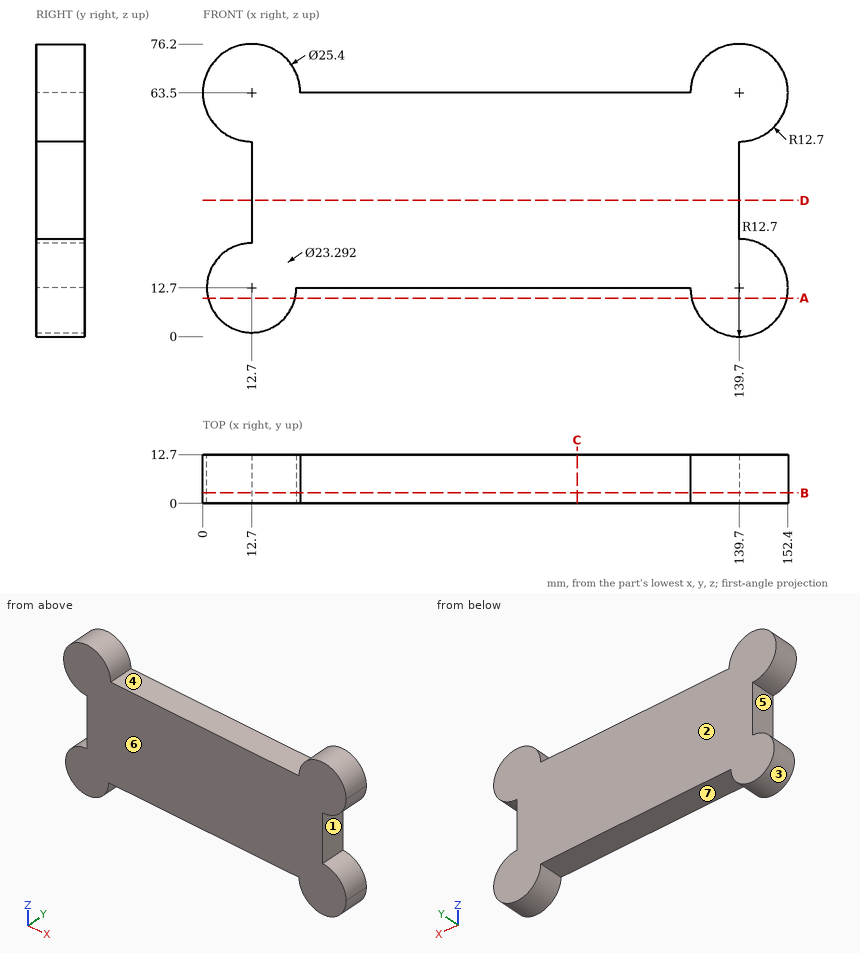
Design review of the part shown in the three views and the two pictorial views. Dimensions are in mm from the part's minimum x, y and z. A direction names the side the tool comes from. Give positions to 0.01 mm unless a question says otherwise; leave off trailing zeros. Loops run counter-clockwise (first coordinate to the right, second up) from the corner with the lowest first, then second, coordinate; pieces in that order, holes last. Notation, with made-up numbers: (49.5, 36.25) -> (101.5, 36.25) arc R33 ccw to (101.5, 64.25) -> close; hole circle Ø11 at (28.25, 13). An arc over 180 degrees is marked (long way). One line per item, written item: value.
Q1. For pin 1 Ø5 at (y, z) = (7.5, 49.5) entering from +X; pin 2 Ø1.5 at (x, y) = (60.5, 6) entering from -Z; pin 3 Ø6.5 at (y, z) = (6, 39.5) entering from -X, all flat-tipped, find the tip position at first contact; note any pin that passes through.
Numbers:
pin 1: stops at x = 145.09
pin 2: stops at z = 12.7
pin 3: stops at x = 12.7
Q2. We need section B-B on y = 2.75. Give the boundary of the cut face in (x, z), and give its area (3 significant figures).
Numbers:
outline: (12.7, 24.35) arc R11.65 ccw (long way) to (24.35, 12.7) -> (127, 12.7) arc R12.7 ccw (long way) to (139.7, 25.4) -> (139.7, 50.8) arc R12.7 ccw (long way) to (127, 63.5) -> (25.4, 63.5) arc R12.7 ccw (long way) to (12.7, 50.8) -> close
area: 7,910 mm^2
Q3. We need section D-D on z = 35.5. Give the boundary of the cut face in (x, y), and give its area (3 significant figures).
Numbers:
outline: (12.7, 0) -> (139.7, 0) -> (139.7, 12.7) -> (12.7, 12.7) -> close
area: 1,610 mm^2
Q4. We need section C-C on x = 97.5. Give the boundary of the cut face in (y, z), and give its area (3 significant figures).
Numbers:
outline: (0, 12.7) -> (12.7, 12.7) -> (12.7, 63.5) -> (0, 63.5) -> close
area: 645 mm^2
Q5. For L1, parallel to X at y = 4, z = 38.5; L2, parallel to Z at x = 69.5, y = 4.25; L3, parallel to X at y = 3, z = 70.5, list the stretches that pass through material, from the lowest coordinate up.
Numbers:
L1: x = 12.7 to 139.7
L2: z = 12.7 to 63.5
L3: x = 2.1 to 23.3, 129.1 to 150.3
Q6. Machinability: for the marked faces 5, 6 and 7, which of the approach directions +Z, -Z, +X, -X, +Y, -Y give a long, thin tool a straight path to every point of the face, cutting with its end or side? Answer none if there is none.
Numbers:
face 5: -X, +Y, -Y
face 6: +Z, -Z, +X, -X, -Y
face 7: -Z, +Y, -Y
Q7. We need section A-A on z = 10. Give the boundary of the cut face in (x, y), and give its area (3 significant figures).
Numbers:
outline: (1.37, 0) -> (24.03, 0) -> (24.03, 12.7) -> (1.37, 12.7) -> close; (127.29, 0) -> (152.11, 0) -> (152.11, 12.7) -> (127.29, 12.7) -> close
area: 603 mm^2
Q8. Draft analysis for pull direction X (two halves, no side actions). For the marked faces 1, 2, 3 and 4, state which applies: pulls with the +X half, pulls with the -X half, needs draft (parallel to the pull), parting line crosses it, or undercut.
Numbers:
face 1: pulls with the +X half
face 2: needs draft
face 3: undercut
face 4: undercut
